Read the model definition and answer for the solid it produces. Units are mm, in the model's axes. A direction names the side the tool comes from. Coordinates: 2 decimals unless noted, no trailing zeros. Loops run counter-clockwise (first coordinate to the right, second up) from the corner with the lowest first, then second, coordinate; pieces in that order, holes last.
Q1. The mould has two halves that part along X. Classify faces 6 (the face through (0.209, -12.522, 39.692)), 7 (the face through (0, -18, 50.8)), 8 (the face through (-8.004, -19.317, 49.321)): pulls with the +X half, pulls with the -X half, needs draft (parallel to the pull), parting line crosses it, or undercut.
Q2. Flat-ended cylindrical pins translate along their axes: P1, Ø9.5, axis at x = 2.5, z = -39, coming from the -Y side (3 decimals); P2, Ø4, axis at x = -6, y = -33, coming from the -Z side; P3, Ø5.5, axis at x = 1.5, z = -16, coming from the -Y side (3 decimals). Find the tip coordinate at first contact, or state that the pin passes through.
Q3. Section A-A (y = -21) is taken. Count the separate pieces of the cut face and the enclosed holes in it, then the cut area to 3 significant figures.
Q4. Straight lines are drawn through the part: line 1 (X direction, y = -13.75, z = 44.45) (1 decimal); line 2 (X direction, y = -29.25, z = 44.45) (3 decimals); line 3 (Y direction, x = -4, z = -4.5) (3 decimals). For each, find the intervals that lie inside material, in ascending order.
Q5. Which of the six approach directions +Z, -Z, +X, -X, +Y, -Y give full straight-line access (tool end or side, diameter ignored) to faces 1 (the face through (0.95, -29.78, 28.43)), 2 (the face through (0.209, -12.522, 20.642)), 3 (the face through (-8.004, -22.298, 20.529)), 4 (the face through (-7.553, -1.565, -48.772)), 5 (the face through (8.046, -22.298, 20.571))?
Q6. Section D-D (z = 25.5) is taken. Give the vertices of the cut face in (x, y) (3 decimals), then the cut area to 3 significant figures.
from build123d import *

# Parameters (mm, degrees)
SKETCH1_W           = 19.05
SKETCH1_H           = 31.75
SKETCH1_R           = 3.175
BOSS_EXTRUDE1_DEPTH = 38.1
SKETCH1_8_R         = 3.175
BOSS_EXTRUDE4_DEPTH = 3.175
SKETCH2_R           = 4.7625
CUT_EXTRUDE1_DEPTH  = 25.4
CHAMFER1_SIZE       = 5
CHAMFER2_SIZE       = 3
SKETCH3_R           = 10.67
CUT_EXTRUDE2_DEPTH  = 109.92610167
SKETCH6_R           = 3.81
CUT_EXTRUDE3_DEPTH  = 5.175
BOSS_EXTRUDE6_START = 1
SKETCH6_3_R         = 5.81
SKETCH6_3_R_2       = 3.81
BOSS_EXTRUDE6_DEPTH = 1
CHAMFER3_SIZE       = 1


with BuildPart() as part:
    # Sketch1 → Boss-Extrude1 (new body)
    with BuildSketch(Plane(origin=(0, 0, 0), x_dir=(1, 0, 0), z_dir=(0, 1, 0))):
        with Locations((0, -34.925)):
            Rectangle(SKETCH1_W, SKETCH1_H)
        with Locations(Location((0, -44.45, 0), (0, 0, 270))):
            Circle(SKETCH1_R, mode=Mode.SUBTRACT)
        with Locations(Location((0, -25.4, 0), (0, 0, 270))):
            Circle(SKETCH1_R, mode=Mode.SUBTRACT)
    extrude(amount=-BOSS_EXTRUDE1_DEPTH)

    # Sketch1<8> → Boss-Extrude4 (add)
    with BuildSketch(Plane(origin=(0, 0, 0), x_dir=(1, 0, 0), z_dir=(0, 1, 0))):
        Polygon((9.525, -50.8), (-9.525, -50.8), (-9.525, 46.8), (-5.525, 50.8), (5.525, 50.8), (9.525, 46.8), align=None)
        with Locations(Location((0, -25.4, 0), (0, 0, 270))):
            Circle(SKETCH1_8_R, mode=Mode.SUBTRACT)
        with Locations(Location((0, -44.45, 0), (0, 0, 270))):
            Circle(SKETCH1_8_R, mode=Mode.SUBTRACT)
    extrude(amount=-BOSS_EXTRUDE4_DEPTH)

    # Sketch2 → Cut-Extrude1 (cut)
    with BuildSketch(Plane(origin=(0, 0, 0), x_dir=(1, 0, 0), z_dir=(0, 1, 0))):
        with Locations(Location((0, -25.4, 0), (0, 0, 270))):
            Circle(SKETCH2_R)
        with Locations(Location((0, -44.45, 0), (0, 0, 270))):
            Circle(SKETCH2_R)
    extrude(amount=-CUT_EXTRUDE1_DEPTH, mode=Mode.SUBTRACT)

    # Chamfer1
    chamfer1_edges = [part.edges().sort_by_distance(p)[0] for p in [
        (0, -3.175, 19.05),
    ]]
    chamfer(chamfer1_edges, length=CHAMFER1_SIZE)

    # Chamfer2
    chamfer2_edges = [part.edges().sort_by_distance(p)[0] for p in [
        (-9.525, -23.1375, 19.05),
        (9.525, -23.1375, 19.05),
        (9.525, -19.05, 50.8),
        (-9.525, -19.05, 50.8),
        (9.525, -5.675, 16.55),
        (-9.525, -5.675, 16.55),
    ]]
    chamfer(chamfer2_edges, length=CHAMFER2_SIZE)

    # Sketch3 → Cut-Extrude2 (cut, through all)
    with BuildSketch(Plane.XY.offset(50.8)):
        with Locations((0, -44.45)):
            Circle(SKETCH3_R)
    extrude(amount=-CUT_EXTRUDE2_DEPTH, mode=Mode.SUBTRACT)

    # Sketch6 → Cut-Extrude3 (cut)
    with BuildSketch(Plane.XZ.offset(3.175)):
        with Locations(Location((0, -41.275, 0), (0, 0, 270))):
            Circle(SKETCH6_R)
    extrude(amount=-CUT_EXTRUDE3_DEPTH, mode=Mode.SUBTRACT)

    # Sketch6<3> → Boss-Extrude6 (add)
    with BuildSketch(Plane.XZ.offset(3.175).offset(BOSS_EXTRUDE6_START)):
        with Locations(Location((0, -41.275, 0), (0, 0, 90))):
            Circle(SKETCH6_3_R)
        with Locations(Location((0, -41.275, 0), (0, 0, 270))):
            Circle(SKETCH6_3_R_2, mode=Mode.SUBTRACT)
    extrude(amount=-BOSS_EXTRUDE6_DEPTH)

    # Chamfer3
    chamfer3_edges = [part.edges().sort_by_distance(p)[0] for p in [
        (0, -3.175, -47.085),
    ]]
    chamfer(chamfer3_edges, length=CHAMFER3_SIZE - 0.0001)  # a hair under: the kernel refuses the full size


solid = part.part
Numbers:
1. face 6: undercut
1. face 7: needs draft
1. face 8: pulls with the -X half
2. P1: stops at y = -4.175
2. P2: stops at z = 19.05
2. P3: stops at y = -3.175
3. separate pieces: 1
3. enclosed holes: 2
3. area: 444 mm2
4. line 1: x = -9.5 to -4.8, 4.8 to 9.5
4. line 2: x = -9.525 to -3.175, 3.175 to 9.525
4. line 3: y = -3.175 to 0
5. face 1: +Y, -Y
5. face 2: +Y
5. face 3: -Z, -X, -Y
5. face 4: -Z, -X, +Y, -Y
5. face 5: -Z, +X, -Y
6. outline: (-9.525, -38.1) - (-8.575, -38.1) arc R10.67 cw to (-3.173, -34.263) - (-3.173, -25.4) - (-4.761, -25.4) - (-4.761, 0) - (-9.525, 0) - close; (3.173, -34.263) arc R10.67 cw to (8.575, -38.1) - (9.525, -38.1) - (9.525, 0) - (4.761, 0) - (4.761, -25.4) - (3.173, -25.4) - close
6. area: 378 mm2
